```python
from build123d import *

# Parameters (mm, degrees)
F0_W     = 88.4682275355
F0_H     = 90.6854122877
F0_R     = 27.23223306
F1_DEPTH = 50.8
F2_SIZE  = 10.16
F3_T     = -2.54


with BuildPart() as f1:
    # F0 (on Top) → F1 (new body)
    with BuildSketch(Plane.XY):
        with Locations((5.0342325121, -0.9333491325)):
            Rectangle(F0_W, F0_H)
        Circle(F0_R, mode=Mode.SUBTRACT)
    extrude(amount=F1_DEPTH)

    # F2
    f2_edges = [f1.edges().sort_by_distance(p)[0] for p in [
        (5.034233, -46.276055, 50.8),
        (-39.199881, -0.933349, 50.8),
        (5.034233, 44.409357, 50.8),
        (49.268346, -0.933349, 50.8),
    ]]
    chamfer(f2_edges, length=F2_SIZE)

    # F3
    f3_openings = [f1.faces().sort_by_distance(p)[0] for p in [
        (5.034233, -35.13649, 50.8),
    ]]
    offset(amount=F3_T, openings=f3_openings)


solid = f1.part
```
For this review, take the finished solid that the model builds, in its own axes (mm). A direction names the side the tool comes from. Round coordinates to 2 decimals unless told otherwise and drop trailing zeros. Order: outer loops, then holes, each group sorted by start corner. A loop starts at its lowest first (then second) coordinate and runs counter-clockwise, first axis right, second up.
Q1. We need section B-B, the plane x = 0. Give the boundary of the cut face in (y, z), plus the area to 3 significant figures.
Findings below:
outline: (-46.28, 0) - (-27.23, 0) - (-27.23, 50.8) - (-29.77, 50.8) - (-29.77, 2.54) - (-43.74, 2.54) - (-43.74, 39.59) - (-32.52, 50.8) - (-36.12, 50.8) - (-46.28, 40.64) - close; (27.23, 0) - (44.41, 0) - (44.41, 40.64) - (34.25, 50.8) - (30.66, 50.8) - (41.87, 39.59) - (41.87, 2.54) - (29.77, 2.54) - (29.77, 50.8) - (27.23, 50.8) - close
area: 605 mm2
Q2. Wall thickness on line 1 (Y direction, x = 0, z = 27); line 2 (X direction, y = 18, z = 38); line 3 (Y direction, x = -16, z = 20.5): over which ranges is each line inside the solid? List them lowest first.
Findings below:
line 1: y = -46.28 to -43.74, -29.77 to -27.23, 27.23 to 29.77, 41.87 to 44.41
line 2: x = -39.2 to -36.66, -23.71 to -20.44, 20.44 to 23.71, 46.73 to 49.27
line 3: y = -46.28 to -43.74, -25.11 to -22.04, 22.04 to 25.11, 41.87 to 44.41
Q3. We need section C-C, the plane y = -11.5. Give the boundary of the cut face in (x, z), plus the area to 3 significant figures.
Findings below:
outline: (-39.2, 0) - (-24.68, 0) - (-24.68, 50.8) - (-29.04, 50.8) - (-39.2, 40.64) - close; (24.68, 0) - (49.27, 0) - (49.27, 40.64) - (39.11, 50.8) - (35.52, 50.8) - (46.73, 39.59) - (46.73, 2.54) - (27.46, 2.54) - (27.46, 50.8) - (24.68, 50.8) - close; hole (-36.66, 2.54) - (-27.46, 2.54) - (-27.46, 48.79) - (-36.66, 39.59) - close
area: 633 mm2
Q4. Insertion check: P1, Ø1, axis at y = 11.5, z = 41, coming from the +X side; P2, Ø5, axis at y = -31, z = 44, coming from the -X side. Each pin has a flat end and moves straight along its axis. Give the tip position at first contact, or say it passes through.
Findings below:
P1: stops at x = 49.27
P2: stops at x = -38.34
Q5. Machinability: for faces 4 (the flat face through (4, 41.869, 21)), 5 (the flat face through (49.268, -2, 20)), which of the approach directions +Z, -Z, +X, -X, +Y, -Y give a long, thin tool a straight path to every point of the face, cutting with its end or side? Answer none if there is none.
Findings below:
face 4: none
face 5: +Z, -Z, +X, +Y, -Y
Q6. Mouldability with a two-part tool opening along X and no side actions: class faces 1 (the flat face through (-36.66, -2, 21)), 2 (the flat face through (4.415, -41.125, 45.791)), 3 (the flat face through (-34.05, -1.57, 45.79)) as pulls with the +X half, pulls with the -X half, needs draft (parallel to the pull), parting line crosses it, or undercut.
Findings below:
face 1: undercut
face 2: needs draft
face 3: pulls with the -X half
Q7. We need section A-A, the plane z = 12. Give the boundary of the cut face in (x, y).
Findings below:
outline: (-39.2, -46.28) - (49.27, -46.28) - (49.27, 44.41) - (-39.2, 44.41) - close; circle Ø59.54 at (0, 0); hole (-36.66, -43.74) - (46.73, -43.74) - (46.73, 41.87) - (-36.66, 41.87) - close; hole circle Ø54.46 at (0, 0)
Q8. We need section D-D, the plane z = 47.5. Give the boundary of the cut face in (x, y), plus the area to 3 significant figures.
Findings below:
outline: (-32.34, -39.42) - (42.41, -39.42) - (42.41, 37.55) - (-32.34, 37.55) - close; hole (-28.75, -35.82) - (38.82, -35.82) - (38.82, 33.96) - (-28.75, 33.96) - (-28.75, 7.74) arc R29.77 cw (long way) to (-28.75, -7.74) - close; hole circle Ø54.46 at (0, 0)
area: 1,480 mm2
